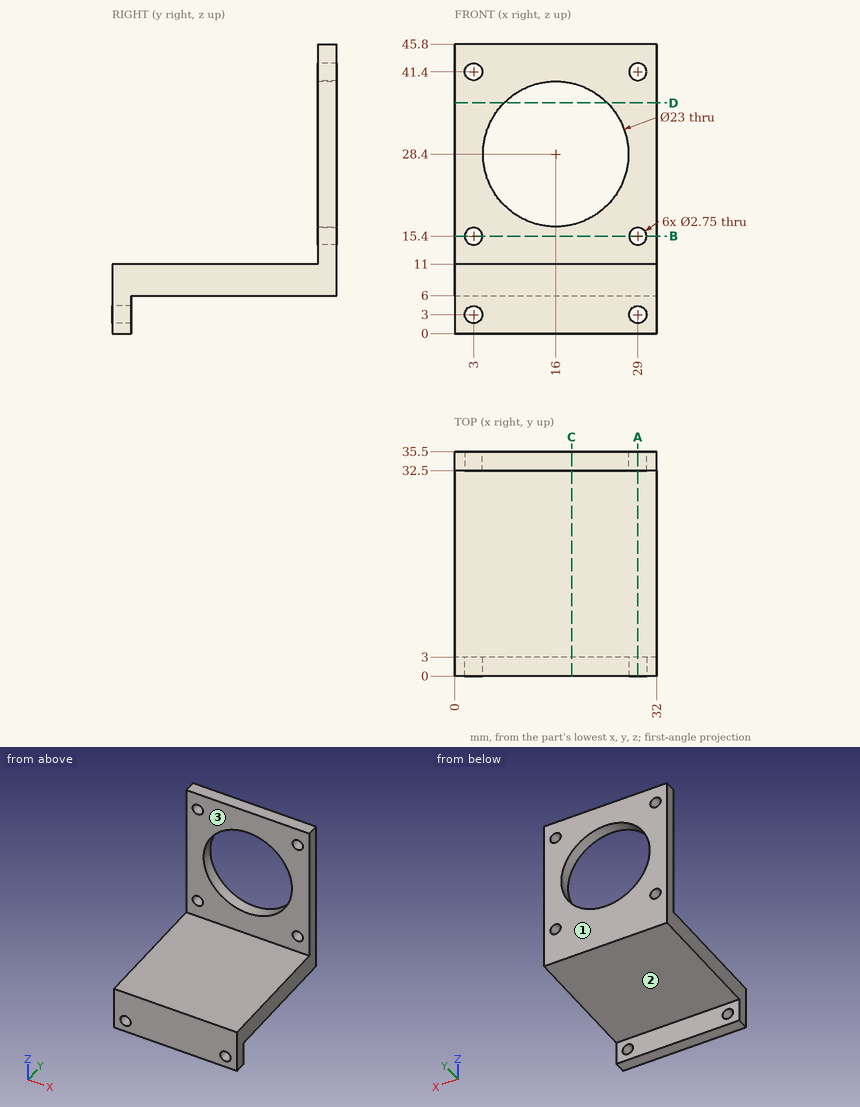
Study the drawing (mm; zero at the part's minimum x, y, z) and answer. A direction names the side the tool comes from. Give positions to 0.01 mm unless a question says otherwise; leave off trailing zeros. Order: outer loops, then holes, each group sorted by start corner. A loop starts at its lowest first (then second) coordinate and runs counter-clockwise, first axis right, second up. Notation, with made-up numbers: (20.25, 20.5) - (47.25, 20.5) arc R20 cw to (47.25, 27.5) - close; hole circle Ø9 at (-30, 3). An arc over 180 degrees is marked (long way). Use one line per item in the form item = value. Start each with the question number.
(1) A cutting plane is placed at B-B, the plane z = 15.4. Write down the section's boundary in (x, y) (3 decimals), then the cut area to 3 significant figures.
(2) For the marked faces 1, 2 and 3, determine the directions among +Z, -Z, +X, -X, +Y, -Y from which every point of the face is accessible in a straight line to the end or side of a thin tool.
(3) A cutting plane is placed at D-D, the plane z = 36.5. Write down the section's boundary in (x, y), then the cut area to 3 significant figures.
(4) A cutting plane is placed at A-A, the plane x = 29. Write down the section's boundary in (y, z) (3 decimals), then the cut area to 3 significant figures.
(5) A cutting plane is placed at C-C, the plane x = 18.5. Write down the section's boundary in (y, z).
(6) Flat-ended cylindrical pins translate along their axes: pin 1 Ø8 at (x, y) = (17.5, 8.5) entering from +Z; pin 2 Ø12 at (x, y) = (14, 9.5) entering from -Z; pin 3 Ø1 at (y, z) = (30.5, 39.5) entering from +X; pin 4 Ø4.5 at (x, z) = (29, 41.4) entering from -Y. Find the tip coordinate at first contact, or state that the pin passes through.
(7) Consider line 1 (Z direction, x = 3, y = 34.7) (3 decimals); line 2 (Z direction, x = 16, y = 34); line 3 (X direction, y = 34, z = 28). Determine where each line is inside the solid, lowest interval first. Write a range as from..to.
Ans:
q1.outline = (0, 32.5) - (1.625, 32.5) - (1.625, 35.5) - (0, 35.5) - close; (4.375, 32.5) - (27.625, 32.5) - (27.625, 35.5) - (4.375, 35.5) - close; (30.375, 32.5) - (32, 32.5) - (32, 35.5) - (30.375, 35.5) - close
q1.area = 79.5 mm^2
q2.face_1 = +Z, -Z, +X, -X, +Y
q2.face_2 = -Z, +X, -X, +Y
q2.face_3 = +Z, +X, -X, -Y
q3.outline = (0, 32.5) - (7.84, 32.5) - (7.84, 35.5) - (0, 35.5) - close; (24.16, 32.5) - (32, 32.5) - (32, 35.5) - (24.16, 35.5) - close
q3.area = 47.0 mm^2
q4.outline = (0, 0) - (3, 0) - (3, 1.625) - (0, 1.625) - close; (0, 4.375) - (3, 4.375) - (3, 6) - (35.5, 6) - (35.5, 14.025) - (32.5, 14.025) - (32.5, 11) - (0, 11) - close; (32.5, 16.775) - (35.5, 16.775) - (35.5, 40.025) - (32.5, 40.025) - close; (32.5, 42.775) - (35.5, 42.775) - (35.5, 45.8) - (32.5, 45.8) - close
q4.area = 275 mm^2
q5.outline = (0, 0) - (3, 0) - (3, 6) - (35.5, 6) - (35.5, 17.18) - (32.5, 17.18) - (32.5, 11) - (0, 11) - close; (32.5, 39.62) - (35.5, 39.62) - (35.5, 45.8) - (32.5, 45.8) - close
q6.pin_1 = 11
q6.pin_2 = 6
q6.pin_3 = through
q6.pin_4 = 32.5
q7.line_1 = 6..14.025, 16.775..40.025, 42.775..45.8
q7.line_2 = 6..16.9, 39.9..45.8
q7.line_3 = 0..4.51, 27.49..32
